```python
from build123d import *

# Parameters (mm, degrees)
F0_W     = 203.2
F0_H     = 31.75
F1_DEPTH = 3.175
F3_D     = 17.145
F4_D     = 4.318


with BuildPart() as f1:
    # F0 (on Right) → F1 (new body)
    with BuildSketch(Plane.YZ):
        Rectangle(F0_W, F0_H)
    extrude(amount=-F1_DEPTH)

    # F3 (through all)
    with Locations(Plane.YZ):
        with Locations((85.725, 0), (53.975, 0)):
            Hole(F3_D / 2)

    # F4 (through all)
    with Locations(Plane.YZ):
        with Locations((-76.50988, 9.17702), (-32.05988, 9.17702)):
            Hole(F4_D / 2)


solid = f1.part
```
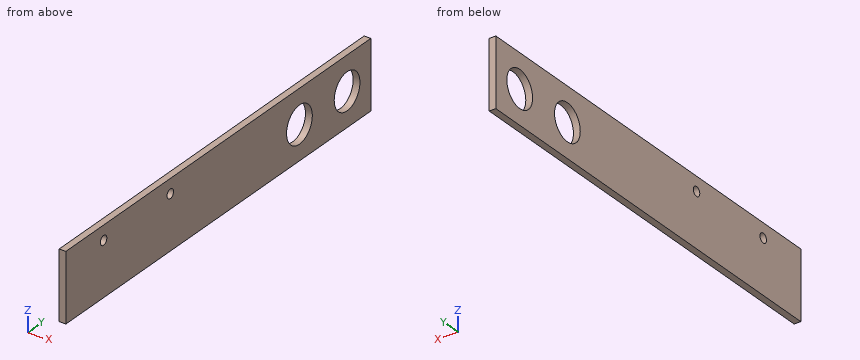
Check sheet for the modelled part. Datum: model origin and axes. Units: mm. Coordinates: 2 decimals unless noted, no trailing zeros. Order: outer loops, then holes, each group sorted by start corner. A loop starts at its lowest first (then second) coordinate and runs counter-clockwise, first axis right, second up. Notation, with made-up numbers: (32, 60) -> (83, 60) arc R21 ccw to (83, 91) -> close; hole circle Ø11 at (-29, 38.25). An arc over 180 degrees is marked (long way). Write each question's results on one line, items separated by ' | '. Start each with the question number.
1) Depth check by flat-ended pin: pin 1 (8 mm diameter, centred on y = 19.5, z = -8, fed in from +X). Enter the tip coordinate at first touch or a pass-through.
2) Section check A-A (z = 0). Enter the section's corners in (x, y) (1 decimal).
3) Section check B-B (x = -2.45). Enter the section's corners in (y, z) (1 decimal), and give its area (3 significant figures).
4) Material ranges on line 1 along Y through (x, z) = (-2.6, -3.5); line 2 along Y through (x, z) = (-0.95, 6); line 3 along Z through (x, y) = (-2.6, 81) (3 decimals), recorded low to high.
Checked values:
1) pin 1: x = 0
2) outline: (-3.2, -101.6) -> (0, -101.6) -> (0, 45.4) -> (-3.2, 45.4) -> close; (-3.2, 62.5) -> (0, 62.5) -> (0, 77.2) -> (-3.2, 77.2) -> close; (-3.2, 94.3) -> (0, 94.3) -> (0, 101.6) -> (-3.2, 101.6) -> close
3) outline: (-101.6, -15.9) -> (101.6, -15.9) -> (101.6, 15.9) -> (-101.6, 15.9) -> close; hole circle Ø4.3 at (-76.5, 9.2); hole circle Ø4.3 at (-32.1, 9.2); hole circle Ø17.1 at (54, 0); hole circle Ø17.1 at (85.7, 0) | area: 5,960 mm²
4) line 1: -101.6 to 46.15, 61.8 to 77.9, 93.55 to 101.6 | line 2: -101.6 to 47.85, 60.1 to 79.6, 91.85 to 101.6 | line 3: -15.875 to -7.153, 7.153 to 15.875
